Verification items for the finished model (mm, model axes). A direction names the side the tool comes from. Give positions to 0.01 mm unless a question says otherwise; leave off trailing zeros. Order: outer loops, then holes, each group sorted by start corner. A loop starts at its lowest first (then second) coordinate and runs counter-clockwise, first axis right, second up. Notation, with made-up numbers: (59.5, 16) -> (97.5, 16) arc R26 cw to (97.5, 53) -> close; hole circle Ø5 at (-4, 6). An arc over 180 degrees is marked (long way). Write each question's results on one line, items separated by ' | '. Start each with the question number.
1. Cross-section at A-A, the plane y = 9. Enter the section's corners in (x, z).
2. Cross-section at B-B, the plane x = 33. Enter the section's corners in (y, z), then the cut area to 3 significant figures.
3. Cross-section at C-C, the plane z = -69.5. Enter the section's corners in (x, y), then the cut area to 3 significant figures.
4. Depth check by flat-ended pin: pin 1 Ø6 at (y, z) = (12, -44.5) entering from -X; pin 2 Ø1.3 at (x, y) = (55.5, 4) entering from -Z; pin 3 Ø1.4 at (y, z) = (6, -147) entering from +X. Enter the tip coordinate at first touch or a pass-through.
5. Material ranges on L1, parallel to X at y = 3.25, z = -146; L2, parallel to Y at x = 180, z = -76.5; L3, parallel to X at y = 7.5, z = -39, recorded low to high. Write a range as from..to.
6. Mould release check, pull along Y, two halves, no side actions. Record for faces 1 (the face through (231, 15.748, -42)), 2 (the face through (57, 5.08, -151)), 3 (the face through (234.95, 9, -42)), 4 (the face through (132, 0, -90)): +Y half, -Y half, draft (parallel to the pull), parting line (faces both ways), or undercut.
7. Set-up check for faces 5 (the face through (227.33, 9, -42)), 6 (the face through (57, 6.35, -151)): record each of +Z, -Z, +X, -X, +Y, -Y from which the full face is reachable in a straight line by a thin tool's end or side.
from build123d import *

# Parameters (mm, degrees)
SKETCH4_W           = 228.6
SKETCH4_H           = 139.7
BOSS_EXTRUDE3_DEPTH = 2.54
SKETCH5_W           = 33.02
SKETCH5_H           = 5.08
BOSS_EXTRUDE4_DEPTH = 2.54
SKETCH6_W           = 40.64
SKETCH6_H           = 27.94
BOSS_EXTRUDE5_DEPTH = 1.27
BOSS_EXTRUDE7_DEPTH = 13.208
FILLET1_R           = 2.54


with BuildPart() as part:
    # Sketch4 → Boss-Extrude3 (new body)
    with BuildSketch(Plane(origin=(0, 0, 0), x_dir=(1, 0, 0), z_dir=(0, 1, 0))):
        with Locations((133.35, 88.9)):
            Rectangle(SKETCH4_W, SKETCH4_H)
    extrude(amount=BOSS_EXTRUDE3_DEPTH)

    # Sketch5 → Boss-Extrude4 (add)
    with BuildSketch(Plane(origin=(0, 2.54, 0), x_dir=(1, 0, 0), z_dir=(0, 1, 0))):
        with Locations((57.15, 146.05)):
            Rectangle(SKETCH5_W, SKETCH5_H)
    extrude(amount=BOSS_EXTRUDE4_DEPTH)

    # Sketch6 → Boss-Extrude5 (add)
    with BuildSketch(Plane(origin=(0, 5.08, 0), x_dir=(1, 0, 0), z_dir=(0, 1, 0))):
        with Locations((57.15, 151.13)):
            Rectangle(SKETCH6_W, SKETCH6_H)
    extrude(amount=BOSS_EXTRUDE5_DEPTH)

    # Sketch8 → Boss-Extrude7 (add)
    with BuildSketch(Plane(origin=(0, 2.54, 0), x_dir=(1, 0, 0), z_dir=(0, 1, 0))):
        Polygon((227.33, 49.53), (234.95, 52.07), (234.95, 31.75), (227.33, 34.29), align=None)
    extrude(amount=BOSS_EXTRUDE7_DEPTH)

    # Fillet1
    fillet1_edges = [part.edges().sort_by_distance(p)[0] for p in [
        (227.33, 9.144, -49.53),
        (227.33, 9.144, -34.29),
        (234.95, 9.144, -31.75),
        (234.95, 9.144, -52.07),
    ]]
    fillet(fillet1_edges, radius=FILLET1_R)


solid = part.part
Results below:
1) outline: (227.33, -47.7) arc R2.54 ccw to (229.07, -50.11) -> (231.61, -50.96) arc R2.54 ccw to (234.95, -48.55) -> (234.95, -35.27) arc R2.54 ccw to (231.61, -32.86) -> (229.07, -33.71) arc R2.54 ccw to (227.33, -36.12) -> close
2) outline: (0, -158.75) -> (2.54, -158.75) -> (2.54, -19.05) -> (0, -19.05) -> close | area: 355 mm²
3) outline: (19.05, 0) -> (247.65, 0) -> (247.65, 2.54) -> (19.05, 2.54) -> close | area: 581 mm²
4) pin 1: stops at x = 227.33 | pin 2: stops at z = -148.59 | pin 3: stops at x = 77.47
5) L1: x = 40.64..73.66 | L2: y = 0..2.54 | L3: x = 227.33..234.95
6) face 1: +Y half | face 2: undercut | face 3: draft | face 4: -Y half
7) face 5: +Z, -Z, -X, +Y | face 6: +Z, -Z, +X, -X, +Y
